Autodesk Inventor part; units mm, degrees
ref_plane "YZ Plane" through (0, 0, 0) normal (1, 0, 0) x (0, 1, 0)
ref_plane "XZ Plane" through (0, 0, 0) normal (0, 1, 0) x (-1, 0, 0)
ref_plane "XY Plane" through (0, 0, 0) normal (0, 0, 1) x (1, 0, 0)
sketch "Sketch1" plane through (0, 0, 0) normal (0, 1, 0) x (-1, 0, 0)
  line L0 (145, -100) -> (-145, -100)
  line L1 (-145, -100) -> (-145, 100)
  line L2 (-145, 100) -> (145, 100)
  line L3 (145, 100) -> (145, -100)
  line L4 (210, 0) -> (-210, 0)
  line L5 (0, -140) -> (0, 140)
  point P0 (0, 0)
  dimension "d30" = 290
  dimension "d31" = 200
extrude "Extrusion1" add sketch "Sketch1" along normal blind 6
sketch "Sketch2" plane through (0, 6, 0) normal (0, 1, 0) x (1, 0, 0)
  circle A0 centre (-19.75, -29.5) radius 13.5
  circle A1 centre (-82.75, -9.5) radius 13.5
  circle A2 centre (-19.75, 9.5) radius 13.5
  circle A3 centre (46.75, 29.5) radius 13.5
  circle A4 centre (82.75, 20.5) radius 13.5
  circle A5 centre (10.75, 29.5) radius 13.5
  circle A6 centre (10.75, -9.5) radius 13.5
  circle A7 centre (46.75, -9.5) radius 13.5
  circle A8 centre (82.75, -18.5) radius 13.5
  line L0 (-96.25, 43) -> (96.25, 43)
  line L1 (96.25, 43) -> (96.25, -43)
  line L2 (96.25, -43) -> (-96.25, -43)
  line L3 (-96.25, -43) -> (-96.25, 43)
  line L4 (145, 100) -> (-145, 100)
  line L5 (145, -100) -> (145, 100)
  line L6 (0, 140) -> (0, -140)
  line L7 (-210, 0) -> (210, 0)
  line L8 (-102.75, 31.5) -> (-62.75, 31.5)
  line L9 (-62.75, 31.5) -> (-62.75, -50.5)
  line L10 (-62.75, -50.5) -> (-102.75, -50.5)
  line L11 (-102.75, -50.5) -> (-102.75, 31.5)
  circle A9 centre (-102.75, 31.5) radius 2.5
  circle A10 centre (-62.75, 31.5) radius 2.5
  circle A11 centre (-102.75, -50.5) radius 2.5
  circle A12 centre (-62.75, -50.5) radius 2.5
  dimension "d3" = 27
  dimension "d19" = 30.5
  dimension "d20" = 36
  dimension "d23" = 19
  dimension "d24" = 9
  dimension "d25" = 36
  dimension "d26" = 11
  dimension "d27" = 9
  dimension "d28" = 11
  dimension "d29" = 63
  dimension "d35" = 41
  dimension "d36" = 41
  dimension "d37" = 20
  dimension "d38" = 20
  dimension "d39" = 5
  dimension "d40" = 5
  dimension "d41" = 5
  dimension "d42" = 5
extrude "Extrusion2" cut sketch "Sketch2" against normal blind 30 contours A0 | A8 | L6 A6 L7 | A6 L6 | A12 L10 L9 | L9 L10 A12 | A1 L7 | L7 A1 | L7 A2 | A2 L7 | A10 L8 L9 | L9 L8 A10 | A4 | A3 | A6 L7 | A11 L11 L10 | L10 L11 A11 | L7 A7 | A7 L7 | L6 A5 | A5 L6 | A9 L11 L8 | L8 L11 A9 picked at (6.7806, -6.3333)
fillet "Fillet1" radius 5 4 edges at (-145, 3, 100) (145, 3, 100) (145, 3, -100) (-145, 3, -100)
sketch "Sketch3" plane through (0, 6, 0) normal (0, 1, 0) x (1, 0, 0)
  circle A0 centre (-139.6667, 94.6667) radius 1.5
  line L0 (140, 100) -> (-140, 100)
  line L1 (-145, 95) -> (-145, -95)
  point P0 (0, 0)
  dimension "d43" = 5.3333
  dimension "d44" = 5.3333
  dimension "d53" = 3
extrude "Extrusion3" cut sketch "Sketch3" against normal blind 20
pattern_linear "Rectangular Pattern1" count 2 spacing 279.3333 along (1, 0, 0) count 2 spacing 189.3333 along (0, 0, 1) of "Extrusion3"
equation "\"d30\" = BoxLength"
equation "\"d31\" = BoxWidth"
equation "\"d3\" = JS_Hole_dia"
equation "\"d36\" = 0.5 * JS_SH_L"
equation "\"d37\" = 0.5 * JS_SH_W"
equation "\"d38\" = 0.5 * JS_SH_W"
equation "\"d39\" = JS_SH_dia"
equation "\"d40\" = JS_SH_dia"
equation "\"d41\" = JS_SH_dia"
equation "\"d42\" = JS_SH_dia"
equation "\"d34\" = CornerOffset"
equation "\"d43\" = 0.666667 * CornerOffset + 0.333333 * SheetThickness"
equation "\"d44\" = 0.666667 * CornerOffset + 0.333333 * SheetThickness"
equation "\"d49\" = BoxLength - 1.33333 * CornerOffset - 0.666667 * SheetThickness"
equation "\"d52\" = BoxWidth - 1.33333 * CornerOffset - 0.666667 * SheetThickness"
equation "\"BoxLength\" = 290"
equation "\"BoxWidth\" = 200"
equation "\"JS_SH_L\" = 82"
equation "\"JS_SH_dia\" = 5"
equation "\"SheetThickness\" = 6"
equation "\"CornerOffset\" = 5"
equation "\"NutS\" = 5.7"
equation "\"NutThreadD2\" = 4.17"
equation "\"SideNutWidth\" = 2.5"
equation "\"JS_Hole_dia\" = 27"
properties part number "sega_straight"
Could you check a few things on this model? Use its own coordinates, in mm. Give positions to 0.01 mm unless a question says otherwise; leave off trailing zeros. Loops run counter-clockwise (first coordinate to the right, second up) from the corner with the lowest first, then second, coordinate; pieces in that order, holes last. Notation, with made-up numbers: M 57.5,88.5 L 65.5,88.5 A22 ccw 65.5,105.5 Z; hole C -10.5,4 d6. An arc over 180 degrees is marked long. Answer as a JSON object with one key per item and string values.
Q1. If I drill on probe 1 along Z at (x, y) = (-102.75, 4.65); probe 2 along X at (y, z) = (4.1, 15.5); probe 3 along X at (y, z) = (2.7, -24.5), over which ranges is the centre line in solid material (lowest first)? Write a range as [from, to].
Values found:
{"probe 1": "z = [-100, -34], [-29, 48], [53, 100]", "probe 2": "x = [-145, -94.84], [-70.66, -1.34], [22.84, 34.66], [58.84, 69.59], [95.91, 145]", "probe 3": "x = [-145, -1.79], [23.29, 34.21], [59.29, 69.86], [95.64, 145]"}
Q2. Suppose I cut it at C-C, the plane y = 4.5. State how many separate pieces and enclosed holes the cut face has, plus the area to 3 significant figures.
Values found:
{"separate pieces": "1", "enclosed holes": "17", "area": "52,700 mm²"}
Q3. If we mould it in two halves opening along Z, with no side actions, what happens to faces 1 (the cylindrical face through (69.263, 3.042, -21.094)), 2 (the flat face through (-2, 3, -100)), 3 (the flat face through (2, 3, 100)), 4 (the flat face through (-145, 3, 1))? For each: pulls with the +Z half, pulls with the -Z half, needs draft (parallel to the pull), parting line crosses it, or undercut.
Values found:
{"face 1": "undercut", "face 2": "pulls with the -Z half", "face 3": "pulls with the +Z half", "face 4": "needs draft"}
Q4. Suppose I cut it at D-D, the plane z = 9.5. List the corners of the cut face in (x, y) for me.
Values found:
{"outline": "M -145,0 L -96.25,0 L -96.25,6 L -145,6 Z; M -69.25,0 L -2.75,0 L -2.75,6 L -69.25,6 Z; M 24.25,0 L 33.25,0 L 33.25,6 L 24.25,6 Z; M 60.25,0 L 72.69,0 L 72.69,6 L 60.25,6 Z; M 92.81,0 L 145,0 L 145,6 L 92.81,6 Z"}
Q5. For P1, Ø21.5, axis at x = 82.75, z = 18.5, coming from the -Y side; P2, Ø6.5, axis at x = -62.75, z = 50.5, coming from the -Y side, each with a flat end and sliding along its axis, tell me the tip position at first contact or that it passes through.
Values found:
{"P1": "passes through", "P2": "stops at y = 0"}
Q6. Suppose I cut it at A-A, the plane x = 82.75. List the corners of the cut face in (y, z) for me.
Values found:
{"outline": "M 0,-100 L 6,-100 L 6,-34 L 0,-34 Z; M 0,-7 L 6,-7 L 6,5 L 0,5 Z; M 0,32 L 6,32 L 6,100 L 0,100 Z"}
Q7. Suppose I cut it at B-B, the plane x = -82.75. List the corners of the cut face in (y, z) for me, plus the area to 3 significant figures.
Values found:
{"outline": "M 0,-100 L 6,-100 L 6,-4 L 0,-4 Z; M 0,23 L 6,23 L 6,100 L 0,100 Z", "area": "1,040 mm²"}
